Read the model definition and answer for the solid it produces. Units are mm, in the model's axes. A direction names the side the tool comes from. Coordinates: 2 decimals unless noted, no trailing zeros. Order: outer loops, then holes, each group sorted by start corner. A loop starts at its lowest first (then second) coordinate and runs counter-clockwise, first axis right, second up. Notation, with made-up numbers: (12, 40.5) -> (57, 40.5) arc R20 cw to (57, 47.5) -> close; hole circle Ø3 at (-25.75, -7). An arc over 180 degrees is marked (long way). Answer as a JSON object with one key per item and string values. Group by question number.
1) Consider L1, parallel to X at y = 5, z = -38; L2, parallel to Y at x = 69, z = 52.5. Determine where each line is inside the solid, lowest interval first.
2) Determine the mould class of faces 3 (the flat face through (13, 38.1, 1)), 4 (the cylindrical face through (0.69, 3.13, 79.3)), 5 (the cylindrical face through (2.065, 31.523, 31.305)) for opening direction Y: released by +Y, released by -Y, zero draft, split by the parting line, or undercut.
3) A tool of negligible diameter and unlimited length cuts with its end or side. For faces 1 (the flat face through (-60, 6.35, 27)), 2 (the cylindrical face through (-69.02, 3.13, -39.05)), from which of +Z, -Z, +X, -X, +Y, -Y can it reach the whole face along a straight path? Write none if from no direction.
4) Section C-C on x = 0 is taken. Count the separate pieces of the cut face and the enclosed holes in it, and give its area (3 significant figures).
5) Given pin 1 (4 mm diameter, centred on y = 20.5, z = 47, fed in from +X); pin 2 (10 mm diameter, centred on x = -5.5, y = 18.5, fed in from -Z); pin 3 (1.5 mm diameter, centred on x = -7.5, y = 33, fed in from -Z), each flat-ended and moving along its own axis, determine where each tip first touches the part or whether it passes through.
6) Section D-D on z = -49 is taken. Determine the outline of the cut face in (x, y).
from build123d import *

# Parameters (mm, degrees)
F_1_4_0_25_DIAMETER_HOLE1_D = 6.35
CIRPATTERN2_COUNT           = 12
SKETCH6_R                   = 9.525
CUT_EXTRUDE1_DEPTH          = 132.369821496


with BuildPart() as part:
    # Sketch1 → Revolve1 (revolve)
    with BuildSketch(Plane.XY, mode=Mode.PRIVATE) as revolve1_sk:
        with BuildLine():
            Line((7.9375, 38.1), (7.9375, 11.1125))
            ThreePointArc((7.9375, 11.1125), (22.02778747, 2.86649456), (38.1, 0))
            Line((38.1, 0), (88.9, 0))
            Line((88.9, 0), (88.9, 6.35))
            Line((88.9, 6.35), (63.5, 6.35))
            Line((63.5, 6.35), (63.5, 38.1))
            Line((63.5, 38.1), (7.9375, 38.1))
        make_face()
    revolve(revolve1_sk.sketch.rotate(Axis((0, 0, 0), (0, 1, 0)), 90), axis=Axis((0, 0, 0), (0, 1, 0)))

    # 1/4 (0.25) Diameter Hole1 (through all)
    with Locations(Plane(origin=(0, 6.35, 0), x_dir=(1, 0, 0), z_dir=(0, 1, 0))):
        with Locations((0, -76.2)):
            f_1_4_0_25_diameter_hole1 = Hole(F_1_4_0_25_DIAMETER_HOLE1_D / 2)

    # CirPattern2: 1/4 (0.25) Diameter Hole1 ×12 about axis, 1 skipped
    cirpattern2_axis = Axis((0, 0, 0), (0, 1, 0))
    add([f_1_4_0_25_diameter_hole1.rotate(cirpattern2_axis, i * 360 / CIRPATTERN2_COUNT) for i in range(1, CIRPATTERN2_COUNT) if i not in (11,)], mode=Mode.SUBTRACT)

    # Sketch6 → Cut-Extrude1 (cut, through all)
    with BuildSketch(Plane.XY):
        with Locations(Location((0, 22.225, 0), (0, 0, 180))):
            Circle(SKETCH6_R)
    extrude(amount=CUT_EXTRUDE1_DEPTH, mode=Mode.SUBTRACT)


solid = part.part
Worked answers:
{
 "1": {"L1": "x = -80.37 to -69.16, -62.82 to 62.82, 69.16 to 80.37", "L2": "y = 0 to 6.35"},
 "2": {"face 3": "released by +Y", "face 4": "zero draft", "face 5": "undercut"},
 "3": {"face 1": "+Y", "face 2": "+Y, -Y"},
 "4": {"separate pieces": "5", "enclosed holes": "0", "area": "3,210 mm²"},
 "5": {"pin 1": "stops at x = 44.8", "pin 2": "stops at z = -63.5", "pin 3": "stops at z = -63.14"},
 "6": {"outline": "(-74.18, 0) -> (74.18, 0) -> (74.18, 6.35) -> (40.39, 6.35) -> (40.39, 38.1) -> (-40.39, 38.1) -> (-40.39, 6.35) -> (-74.18, 6.35) -> close"}
}
